Source: CAD feature listing. Evaluate the final solid. Frame: model axes, mm. Face numbers are marked on the shaded views. A direction names the side the tool comes from. Coordinates: 2 decimals unless noted, no trailing zeros. Loops run counter-clockwise (first coordinate to the right, second up) from the corner with the lowest first, then second, coordinate; pieces in that order, holes last.
```python
from build123d import *

# Parameters (mm, degrees)
F0_W     = 40
F0_H     = 40
F0_R     = 1.75
F1_DEPTH = 10
F2_R     = 3
F3_DEPTH = 3.5
F5_DEPTH = 3
F6_R     = 1.25
F7_DEPTH = 10.001


with BuildPart() as f1:
    # F0 (on Top) → F1 (new body)
    with BuildSketch(Plane.XY):
        Rectangle(F0_W, F0_H)
        with Locations((0, -15)):
            Circle(F0_R, mode=Mode.SUBTRACT)
        with Locations((-15, 0)):
            Circle(F0_R, mode=Mode.SUBTRACT)
        with Locations((15, 0)):
            Circle(F0_R, mode=Mode.SUBTRACT)
        with Locations((0, 15)):
            Circle(F0_R, mode=Mode.SUBTRACT)
    extrude(amount=F1_DEPTH)

    # F2 (on face) → F3 (cut)
    with BuildSketch(Plane.XY.offset(10)):
        with Locations((-15, 0)):
            Circle(F2_R)
        with Locations((0, 15)):
            Circle(F2_R)
        with Locations((15, 0)):
            Circle(F2_R)
        with Locations((0, -15)):
            Circle(F2_R)
    extrude(amount=-F3_DEPTH, mode=Mode.SUBTRACT)

    # F4 (on face) → F5 (cut)
    with BuildSketch(Plane(origin=(0, 0, 0), x_dir=(1, 0, 0), z_dir=(0, 0, -1))):
        Polygon((4.242641, -18.384776), (18.384776, -4.242641), (-4.242641, 18.384776), (-18.384776, 4.242641), align=None)
    extrude(amount=-F5_DEPTH, mode=Mode.SUBTRACT)

    # F6 (on face) → F7 (cut, through all)
    with BuildSketch(Plane(origin=(0, 0, 0), x_dir=(1, 0, 0), z_dir=(0, 0, -1))):
        with Locations((0, 12.020815)):
            Circle(F6_R)
        with Locations((12.020815, 0)):
            Circle(F6_R)
        with Locations((-12.020815, 0)):
            Circle(F6_R)
        with Locations((0, -12.020815)):
            Circle(F6_R)
    extrude(amount=-F7_DEPTH, mode=Mode.SUBTRACT)


solid = f1.part
```
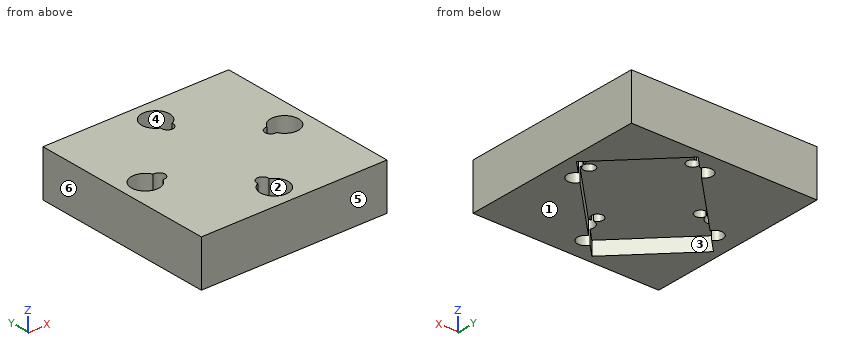
Q1. Material intervals for line 1 along Y through (x, z) = (0, 5.75); line 2 along X through (y, z) = (-12, 8.25); line 3 along X through (y, z) = (2, 8), sorted ascending.
Q2. Section query D-D on z = 5.25. Return the cut outline in (x, y), then the cut area to 3 significant figures.
Q3. Draft query along Y for the marked faces 4, 5 and 6. Return one class per face: released by +Y, released by -Y, zero draft, split by the parting line, or undercut.
Q4. Section query A-A on x = -15. Return the cut outline in (y, z).
Q5. Reachability of the marked faces 1, 2 and 3 from +Z, -Z, +X, -X, +Y, -Y: full face, straight path, thin tool, end or side. Return the list, or none.
Q6. Section query C-C on x = 6. Return the cut outline in (y, z), then the cut area to 3 significant figures.
Q7. First-contact query: pin 1 Ø8 at (x, y) = (-15, 0) entering from -Z; pin 2 Ø3 at (x, y) = (-14, 0) entering from +Z; pin 3 Ø1.5 at (x, y) = (12.02, 0) entering from +Z; pin 4 Ø1.5 at (x, y) = (3, 3.5) entering from -Z. Flat tips, straight axial feed; report the tip coordinate or a pass-through.
Q8. Section query B-B on y = 15. Return the cut outline in (x, z), then the cut area to 3 significant figures.
Resolved:
1. line 1: y = -20 to -16.75, -10.77 to 10.77, 16.75 to 20
1. line 2: x = -20 to -1.25, 1.25 to 20
1. line 3: x = -20 to -17.24, -12.76 to 12.76, 17.24 to 20
2. outline: (-20, -20) - (20, -20) - (20, 20) - (-20, 20) - close; hole (-13.26, -0.17) arc R1.25 ccw (long way) to (-13.26, 0.17) arc R1.75 ccw (long way) to start; hole (-0.17, -13.26) arc R1.75 ccw (long way) to (0.17, -13.26) arc R1.25 ccw (long way) to start; hole (-0.17, 13.26) arc R1.25 ccw (long way) to (0.17, 13.26) arc R1.75 ccw (long way) to start; hole (13.26, -0.17) arc R1.75 ccw (long way) to (13.26, 0.17) arc R1.25 ccw (long way) to start
2. area: 1,540 mm2
3. face 4: undercut
3. face 5: released by -Y
3. face 6: zero draft
4. outline: (-20, 0) - (-7.63, 0) - (-7.63, 3) - (-1.75, 3) - (-1.75, 6.5) - (-3, 6.5) - (-3, 10) - (-20, 10) - close; (1.75, 0) - (20, 0) - (20, 10) - (3, 10) - (3, 6.5) - (1.75, 6.5) - close
5. face 1: -Z, +X, -X, +Y, -Y
5. face 2: +Z
5. face 3: -Z
6. outline: (-20, 0) - (-8.14, 0) - (-8.14, 3) - (16.63, 3) - (16.63, 0) - (20, 0) - (20, 10) - (-20, 10) - close
6. area: 326 mm2
7. pin 1: stops at z = 0
7. pin 2: stops at z = 6.5
7. pin 3: passes through
7. pin 4: stops at z = 3
8. outline: (-20, 0) - (-1.75, 0) - (-1.75, 6.5) - (-3, 6.5) - (-3, 10) - (-20, 10) - close; (1.75, 3) - (7.63, 3) - (7.63, 0) - (20, 0) - (20, 10) - (3, 10) - (3, 6.5) - (1.75, 6.5) - close
8. area: 339 mm2
